Autodesk Inventor part; units mm, degrees
ref_plane "YZ Plane" through (0, 0, 0) normal (1, 0, 0) x (0, 1, 0)
ref_plane "XZ Plane" through (0, 0, 0) normal (0, 1, 0) x (-1, 0, 0)
ref_plane "XY Plane" through (0, 0, 0) normal (0, 0, 1) x (1, 0, 0)
sketch "Sketch1" plane through (0, 0, 0) normal (0, 1, 0) x (-1, 0, 0)
  line L0 (0, 0) -> (-430, 0)
  line L1 (-430, 0) -> (-430, -40)
  line L2 (-430, -40) -> (0, -40)
  line L3 (0, -40) -> (0, 0)
  dimension "d0" = 430
  dimension "d1" = 40
extrude "Extrusion1" add sketch "Sketch1" along normal blind 60
sketch "Sketch2" plane through (0, 0, 0) normal (0, -1, 0) x (1, 0, 0)
  line L0 (430, 0) -> (430, -40)
  line L1 (430, -40) -> (0, -40)
  line L2 (361.5161, 0) -> (430, 0)
  line L3 (180.1999, -1.7586) -> (180.1999, -32.3586)
  line L4 (215.5999, -1.7586) -> (180.1999, -1.7586)
  line L5 (215.5999, -32.3586) -> (215.5999, -1.7586)
  line L6 (180.1999, -32.3586) -> (215.5999, -32.3586)
  line L7 (215.5999, -1.7586) -> (220.5999, -1.7586)
  line L8 (180.1999, -1.7586) -> (175.1999, -1.7586)
  line L9 (175.1999, -1.7586) -> (175.1999, 0)
  line L10 (430, -40) -> (0, -40)
  line L11 (220.5999, -1.7586) -> (220.5999, 0)
  line L12 (215.5999, -32.3586) -> (215.5999, -35.3586)
  line L13 (215.5999, -32.3586) -> (212.5999, -32.3586) construction
  line L14 (220.5999, 0) -> (175.1999, 0)
  line L15 (175.1999, 0) -> (175.1999, -35.3586)
  line L16 (175.1999, -35.3586) -> (220.5999, -35.3586)
  line L17 (220.5999, -35.3586) -> (220.5999, 0)
  point P0 (0, 0)
  point P1 (430, -40)
  dimension "d4" = 5
  dimension "d5" = 5
  dimension "d7" = 3
  dimension "d8" = 90
extrude "Extrusion2" cut sketch "Sketch2" against normal blind 60
sketch "Sketch4" plane through (0, 60, 0) normal (0, 1, 0) x (1, 0, 0)
  line L0 (220.5999, 0) -> (430, 0)
  line L1 (430, 40) -> (0, 40)
  line L2 (220.5999, 35.3586) -> (220.5999, 0)
  line L3 (175.1999, 0) -> (175.1999, 35.3586)
  line L4 (175.1999, 35.3586) -> (220.5999, 35.3586)
  line L5 (0, 0) -> (175.1999, 0)
  line L6 (300.8442, 17.7835) -> (300.8442, 2.5435)
  line L7 (321.1642, 2.5435) -> (321.1642, 17.7835)
  line L8 (300.8442, 2.5435) -> (321.1642, 2.5435)
  line L9 (321.1642, 17.7835) -> (300.8442, 17.7835)
  line L10 (220.5999, 0) -> (430, 0)
  line L11 (295.5283, 0) -> (327.2819, 0)
  line L12 (327.2819, 0) -> (327.2819, 22.353)
  line L13 (327.2819, 22.353) -> (295.5283, 22.353)
  line L14 (295.5283, 22.353) -> (295.5283, 0)
extrude "Extrusion3" cut sketch "Sketch4" against normal blind 60 contours L14 L13 L12 L0 | L9 L7 L8 L6
properties part number "Cadru_2"
The model under review builds one solid part; all positions refer to its coordinate system, in mm. A direction names the side the tool comes from. Coordinates: 2 decimals unless noted, no trailing zeros. Order: outer loops, then holes, each group sorted by start corner. A loop starts at its lowest first (then second) coordinate and runs counter-clockwise, first axis right, second up. Notation, with made-up numbers: (70.5, 65) -> (121.5, 65) arc R20 cw to (121.5, 72) -> close; hole circle Ø1 at (7, -32.5). An arc over 180 degrees is marked (long way). Answer in a Markdown table with one row per item. Add a question column.
Item 1: To check wall thickness, follow probe 1 along X at (y, z) = (21.5, -2.5); probe 2 along X at (y, z) = (23.5, -27); probe 3 along Z at (x, y) = (212, 43). State the ranges of each line that lie inside material, in increasing order.
Item 2: Clearance check with flat-ended pins moving along their axes: pin 1 (8 mm diameter, centred on x = 189, y = 48, fed in from +Z); pin 2 (11 mm diameter, centred on y = 17, z = -16, fed in from -X); pin 3 (16 mm diameter, centred on x = 311, y = 27.5, fed in from +Z). State where each tip first meets the part, or that it passes through.
Item 3: We need section C-C on x = 191.5. Write out the cut boundary in (y, z).
Item 4: We need section A-A on z = -5.5. Write out the cut boundary in (x, y).
Item 5: We need section B-B on y = 34.5. Write out the cut boundary in (x, z), plus the area to 3 significant figures.
Item 6: Machinability: for faces 1 (the flat face through (218, 0, -37)), 2 (the flat face through (327.282, 30, -11)), which of the approach directions +Z, -Z, +X, -X, +Y, -Y give a long, thin tool a straight path to every point of the face, cutting with its end or side? Answer none if there is none.
Final values:
| question | item | result |
|---|---|---|
| 1 | probe 1 | x = 0 to 175.2, 220.6 to 295.53, 327.28 to 430 |
| 1 | probe 2 | x = 0 to 175.2, 220.6 to 430 |
| 1 | probe 3 | z = -40 to -35.36 |
| 2 | pin 1 | stops at z = -35.36 |
| 2 | pin 2 | stops at x = 0 |
| 2 | pin 3 | stops at z = -22.35 |
| 3 | outline | (0, -40) -> (60, -40) -> (60, -35.36) -> (0, -35.36) -> close |
| 4 | outline | (0, 0) -> (175.2, 0) -> (175.2, 60) -> (0, 60) -> close; (220.6, 0) -> (295.53, 0) -> (295.53, 60) -> (220.6, 60) -> close; (327.28, 0) -> (430, 0) -> (430, 60) -> (327.28, 60) -> close |
| 5 | outline | (0, -40) -> (430, -40) -> (430, 0) -> (327.28, 0) -> (327.28, -22.35) -> (295.53, -22.35) -> (295.53, 0) -> (220.6, 0) -> (220.6, -35.36) -> (175.2, -35.36) -> (175.2, 0) -> (0, 0) -> close |
| 5 | area | 14,900 mm2 |
| 6 | face 1 | +Z, -Z, +X, -X, -Y |
| 6 | face 2 | +Z, +Y, -Y |
